Autodesk Inventor part; units mm, degrees
ref_plane "YZ Plane" through (0, 0, 0) normal (1, 0, 0) x (0, 1, 0)
ref_plane "XZ Plane" through (0, 0, 0) normal (0, 1, 0) x (-1, 0, 0)
ref_plane "XY Plane" through (0, 0, 0) normal (0, 0, 1) x (1, 0, 0)
sketch "Sketch1" plane through (0, 0, 0) normal (0, 0, 1) x (1, 0, 0)
  line L0 (-37.1429, 20.9244) -> (432.7571, 20.9244)
  line L1 (432.7571, 20.9244) -> (432.7571, -112.4256)
  line L2 (432.7571, -112.4256) -> (-37.1429, -112.4256)
  line L3 (-37.1429, -112.4256) -> (-37.1429, 20.9244)
  point P0 (0, 0)
  dimension "d0" = 469.9
  dimension "d1" = 133.35
extrude "Extrusion1" add sketch "Sketch1" along normal blind 3.175
sketch "Sketch2" plane through (432.7571, -112.4256, 0) normal (1, 0, 0) x (0, 0, -1)
  line L0 (0, 133.35) -> (0, 0)
  line L1 (-3.175, 133.35) -> (0, 107.95)
  line L2 (-3.175, 0) -> (0, 22.86)
  line L3 (-3.175, 0) -> (0, 0)
  line L4 (0, 22.86) -> (0, 0)
  point P0 (0, 112.4256)
  dimension "d4" = 25.4
  dimension "d5" = 22.86
extrude "Extrusion3" cut sketch "Sketch2" against normal blind 476.25
sketch "Sketch4" plane through (0, 0, 0) normal (0, 0, -1) x (-1, 0, 0)
  line L0 (-432.7571, -89.5656) -> (37.1429, -89.5656)
  line L1 (37.1429, 20.9244) -> (-432.7571, 20.9244)
  line L2 (-432.7571, 20.9244) -> (-432.7571, -89.5656)
  line L3 (-432.7571, -89.5656) -> (37.1429, -89.5656)
  line L4 (37.1429, -89.5656) -> (37.1429, 20.9244)
  line L5 (37.1429, 20.9244) -> (-432.7571, 20.9244)
  line L6 (-432.7571, 20.9244) -> (-432.7571, -89.5656)
  line L7 (-282.4653, -89.5656) -> (-282.4653, 20.9244)
  line L8 (-132.1735, -89.5656) -> (-132.1735, 20.9244)
  line L9 (18.1183, -89.5656) -> (18.1183, 20.9244)
  line L10 (-282.4653, -89.5656) -> (-312.071, 20.9244)
  line L11 (-432.7571, -89.5656) -> (-403.1514, 20.9244)
  line L12 (-282.4653, -89.5656) -> (-252.8596, 20.9244)
  line L13 (-132.1735, -89.5656) -> (-161.7792, 20.9244)
  line L14 (-132.1735, -89.5656) -> (-102.5678, 20.9244)
  line L15 (18.1183, -89.5656) -> (-11.4874, 20.9244)
  line L16 (18.1183, 20.9244) -> (37.1429, 20.9244)
  line L17 (37.1429, 20.9244) -> (37.1429, -89.5656)
  line L18 (37.1429, -89.5656) -> (18.1183, -89.5656)
  line L19 (18.1183, -89.5656) -> (18.1183, 20.9244)
  point P0 (0, 0)
  dimension "d10" = 150.2918
  dimension "d11" = 150.2918
  dimension "d12" = 150.2918
  dimension "d13" = 15
  dimension "d14" = 15
  dimension "d15" = 15
extrude "Extrusion4" add sketch "Sketch4" along normal blind 3.175 contours L2 L1 L11 | L10 L1 L7 | L7 L1 L12 | L13 L1 L8 | L8 L1 L14 | L15 L1 L9
sketch "Sketch5" plane through (0, 0, 0) normal (0, 0, -1) x (-1, 0, 0)
  line L0 (18.1183, 20.9244) -> (18.1183, -89.5656)
  line L1 (18.1183, -89.5656) -> (37.1429, -89.5656)
  line L2 (37.1429, -89.5656) -> (37.1429, 20.9244)
  line L3 (37.1429, 20.9244) -> (18.1183, 20.9244)
  line L4 (18.1183, 20.9244) -> (37.1429, 20.9244)
  line L5 (37.1429, 20.9244) -> (37.1429, -89.5656)
  line L6 (37.1429, -89.5656) -> (18.1183, -89.5656)
  line L7 (18.1183, -89.5656) -> (18.1183, 20.9244)
  point P0 (0, 0)
sketch "Sketch6" plane through (0, 0, 3.175) normal (0, 0, 1) x (1, 0, 0)
  line L0 (-37.1429, 20.9244) -> (-18.1183, 20.9244)
  line L1 (-18.1183, 20.9244) -> (-18.1183, -89.5656)
  line L2 (-18.1183, -89.5656) -> (-37.1429, -89.5656)
  line L3 (-37.1429, -89.5656) -> (-37.1429, 20.9244)
  point P0 (0, 0)
  dimension "d18" = 110.49
  dimension "d19" = 19.0246
extrude "Extrusion5" add sketch "Sketch6" against normal blind 6.35
sketch "Sketch7" plane through (0, 0, 3.175) normal (0, 0, 1) x (1, 0, 0)
  line L0 (-11.4874, 20.9244) -> (-37.1429, 20.9244)
  line L1 (-18.0929, -33.0506) -> (-37.1429, -33.0506)
  line L2 (-37.1429, -33.0506) -> (-37.1429, -58.4506)
  line L3 (-37.1429, -58.4506) -> (-18.0929, -58.4506)
  line L4 (-18.0929, -58.4506) -> (-18.0929, -33.0506)
  line L5 (-37.1429, -112.4256) -> (-37.1429, 20.9244)
  point P0 (0, 0)
  dimension "d22" = 19.05
  dimension "d23" = 25.4
  dimension "d25" = 0
  dimension "d27" = 133.35
  dimension "d28" = 53.975
extrude "Extrusion6" cut sketch "Sketch7" against normal blind 3.175
sketch "Sketch8" plane through (0, 0, 0) normal (0, 0, 1) x (1, 0, 0)
  line L0 (-18.0929, -58.4506) -> (-18.0929, -33.0506)
  line L1 (-18.0929, -33.0506) -> (-37.1429, -33.0506)
  circle A0 centre (-24.4429, -39.4006) radius 1.5875
  circle A1 centre (-24.4429, -52.1006) radius 1.5875
  point P0 (0, 0)
  dimension "d31" = 3.175
  dimension "d32" = 3.175
  dimension "d33" = 6.35
  dimension "d34" = 12.7
  dimension "d35" = 6.35
extrude "Extrusion7" cut sketch "Sketch8" against normal blind 3.175
properties part number "bottom panel"
The listing builds one solid part. Answer for the finished solid, in the listing's coordinates (mm). A direction names the side the tool comes from. Coordinates: 2 decimals unless noted, no trailing zeros. Loops run counter-clockwise (first coordinate to the right, second up) from the corner with the lowest first, then second, coordinate; pieces in that order, holes last. Notation, with made-up numbers: M 4.25,4 L 31.25,4 A18 cw 31.25,14 Z; hole C 16,58.5 d5. An arc over 180 degrees is marked long. Answer in a Markdown table with one row per item.
1) Find section A-A (y = -9). Determine the outline of the cut face in (x, z) (3 decimals).
Answers below:
| item | result |
|---|---|
| outline | M -37.143,-3.175 L 3.469,-3.175 L 3.469,0 L 110.586,0 L 110.586,-3.175 L 153.761,-3.175 L 153.761,0 L 260.878,0 L 260.878,-3.175 L 304.053,-3.175 L 304.053,0 L 411.17,0 L 411.17,-3.175 L 432.757,-3.175 L 432.757,3.175 L -37.143,3.175 Z |
2) Given pin 1 (1.6 mm diameter, centred on y = -41.5, z = 1.5, fed in from -X); pin 2 (2.5 mm diameter, centred on x = -23, z = -2.5, fed in from -Y); pin 3 (6 mm diameter, centred on x = 158, y = -86, fed in from -Z), each flat-ended and moving along its own axis, determine where each tip first touches the part or whether it passes through.
Answers below:
| item | result |
|---|---|
| pin 1 | x = -18.09 |
| pin 2 | y = -89.57 |
| pin 3 | z = 0 |
3) Find section C-C (x = 355.5). Determine the outline of the cut face in (y, z) (3 decimals).
Answers below:
| item | result |
|---|---|
| outline | M -112.426,3.175 L -89.566,0 L 20.924,0 L 20.924,3.175 Z |
4) Find section D-D (y = 12.5). Determine the outline of the cut face in (x, z) (3 decimals).
Answers below:
| item | result |
|---|---|
| outline | M -37.143,-3.175 L 9.23,-3.175 L 9.23,0 L 104.825,0 L 104.825,-3.175 L 159.522,-3.175 L 159.522,0 L 255.117,0 L 255.117,-3.175 L 309.814,-3.175 L 309.814,0 L 405.409,0 L 405.409,-3.175 L 432.757,-3.175 L 432.757,3.175 L -37.143,3.175 Z |
5) Which of the six approach directions +Z, -Z, +X, -X, +Y, -Y give full straight-line access (tool end or side, diameter ignored) to faces 1 (the flat face through (357, -34, 0)), 2 (the flat face through (-28, -46, 0)), 3 (the flat face through (201.1, -101.16, 1.61))?
Answers below:
| item | result |
|---|---|
| face 1 | -Z, -Y |
| face 2 | +Z, -X |
| face 3 | -Z, +X, -X, -Y |
6) Determine the mould class of faces 4 (the flat face through (117.578, -35.094, -1.565)), 5 (the flat face through (133, -21, -3.175)) for opening direction X: released by +X, released by -X, zero draft, split by the parting line, or undercut.
Answers below:
| item | result |
|---|---|
| face 4 | undercut |
| face 5 | zero draft |
7) Find section B-B (z = 1.5). Determine the outline of the cut face in (x, y).
Answers below:
| item | result |
|---|---|
| outline | M -37.14,-100.37 L 432.76,-100.37 L 432.76,20.92 L -37.14,20.92 L -37.14,-33.05 L -18.09,-33.05 L -18.09,-58.45 L -37.14,-58.45 Z |
8) Find the intervals of material crossed by probe 1 along X at (y, z) = (-64.5, -1); probe 2 along X at (y, z) = (-40.5, -3); probe 3 along X at (y, z) = (-68, -1.5), in increasing order.
Answers below:
| item | result |
|---|---|
| probe 1 | -37.14 to -11.4, 125.46 to 138.89, 275.75 to 289.18, 426.04 to 432.76 |
| probe 2 | -37.14 to -25.59, -23.3 to -4.97, 119.03 to 145.32, 269.32 to 295.61, 419.61 to 432.76 |
| probe 3 | -37.14 to -12.34, 126.4 to 137.95, 276.69 to 288.24, 426.98 to 432.76 |
